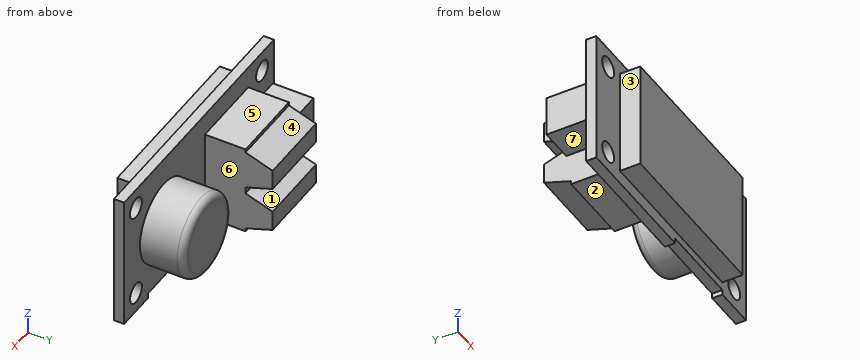
from build123d import *

# Parameters (mm, degrees)
SKETCH1_R           = 1.5
BOSS_EXTRUDE1_DEPTH = 1.5
SKETCH2_R           = 6
BOSS_EXTRUDE2_DEPTH = 6.5
FILLET1_R           = 1
SKETCH3_W           = 5
SKETCH3_H           = 6
BOSS_EXTRUDE3_DEPTH = 6
BOSS_EXTRUDE4_START = -12.5
BOSS_EXTRUDE4_DEPTH = 11
SKETCH6_W           = 26
SKETCH6_H           = 16
BOSS_EXTRUDE5_DEPTH = 3


with BuildPart() as part:
    # Sketch1 → Boss-Extrude1 (new body)
    with BuildSketch(Plane(origin=(0, 0, 0), x_dir=(1, 0, 0), z_dir=(0, 1, 0))):
        Polygon((-19, -10), (19, -10), (19, 10), (13, 10), (13, 9.25), (1, 9.25), (1, 10), (-19, 10), align=None)
        with Locations((-16, 7)):
            Circle(SKETCH1_R, mode=Mode.SUBTRACT)
        with Locations((-16, -7)):
            Circle(SKETCH1_R, mode=Mode.SUBTRACT)
        with Locations((16, -7)):
            Circle(SKETCH1_R, mode=Mode.SUBTRACT)
        with Locations((16, 7)):
            Circle(SKETCH1_R, mode=Mode.SUBTRACT)
    extrude(amount=BOSS_EXTRUDE1_DEPTH)

    # Sketch2 → Boss-Extrude2 (add)
    with BuildSketch(Plane(origin=(0, 1.5, 0), x_dir=(1, 0, 0), z_dir=(0, 1, 0))):
        with Locations((9, 0)):
            Circle(SKETCH2_R)
    extrude(amount=BOSS_EXTRUDE2_DEPTH)

    # Fillet1
    fillet1_edges = [part.edges().sort_by_distance(p)[0] for p in [
        (3, 8, 0),
    ]]
    fillet(fillet1_edges, radius=FILLET1_R)

    # Sketch3 → Boss-Extrude3 (add)
    with BuildSketch(Plane(origin=(0, 1.5, 0), x_dir=(1, 0, 0), z_dir=(0, 1, 0))):
        with Locations((-16.25, 0)):
            Rectangle(SKETCH3_W, SKETCH3_H)
    extrude(amount=BOSS_EXTRUDE3_DEPTH)

    # Sketch5 → Boss-Extrude4 (add)
    with BuildSketch(Plane(origin=(0, 0, 0), x_dir=(0, 0, -1), z_dir=(1, 0, 0)).offset(BOSS_EXTRUDE4_START)):
        Polygon((6.75, 1.5), (6.75, 7.5), (6.25, 7.5), (4.875, 11.5), (1.875, 11.5), (0.5, 7.5), (-0.5, 7.5), (-1.875, 11.5), (-4.875, 11.5), (-6.25, 7.5), (-6.75, 7.5), (-6.75, 1.5), align=None)
    extrude(amount=BOSS_EXTRUDE4_DEPTH)

    # Sketch6 → Boss-Extrude5 (add)
    with BuildSketch(Plane.XZ):
        Rectangle(SKETCH6_W, SKETCH6_H)
    extrude(amount=BOSS_EXTRUDE5_DEPTH)


solid = part.part
Read the model definition and answer for the solid it produces. Units are mm, in the model's axes. Face numbers are marked on the shaded views. A direction names the side the tool comes from. Give positions to 0.01 mm unless a question says otherwise; leave off trailing zeros. Write each loop counter-clockwise with the first axis right and the second up, starting at its lowest first coordinate (ties: lowest second). Pieces come first, ordered by that corner, then holes. Notation, with made-up numbers: (47.25, 11.25) - (64.25, 11.25) arc R27 cw to (64.25, 33.25) - close; hole circle Ø7 at (1.25, -7.75). An arc over 180 degrees is marked (long way). Return JSON: item names as keys, results as strings.
Q1. For a pull along Z with two mould halves and no side action, classify the marked faces 1, 2, 3 and 4 as released by +Z, released by -Z, zero draft, split by the parting line, or undercut.
Reply:
{"face 1": "undercut", "face 2": "released by -Z", "face 3": "zero draft", "face 4": "released by +Z"}
Q2. A cutting plane is placed at D-D, the plane x = 9. Determine the outline of the cut face in (y, z).
Reply:
{"outline": "(-3, -8) - (0, -8) - (0, -9.25) - (1.5, -9.25) - (1.5, -6) - (7, -6) arc R1 ccw to (8, -5) - (8, 5) arc R1 ccw to (7, 6) - (1.5, 6) - (1.5, 10) - (0, 10) - (0, 8) - (-3, 8) - close"}
Q3. A cutting plane is placed at B-B, the plane y = 4.25. Determine the outline of the cut face in (x, z).
Reply:
{"outline": "(-18.75, -3) - (-13.75, -3) - (-13.75, 3) - (-18.75, 3) - close; (-12.5, -6.75) - (-1.5, -6.75) - (-1.5, 6.75) - (-12.5, 6.75) - close; circle Ø12 at (9, 0)"}
Q4. Given P1, Ø2.5, axis at x = 1, y = -2, coming from the +Z side; P2, Ø2.5, axis at y = -2, z = 0.5, coming from the -X side; P3, Ø1.5, axis at x = -15.5, y = 3.5, coming from the -Z side, each flat-ended and moving along its own axis, determine where each tip first touches the part or whether it passes through.
Reply:
{"P1": "z = 8", "P2": "x = -13", "P3": "z = -3"}
Q5. A cutting plane is placed at A-A, the plane x = 16. Determine the outline of the cut face in (y, z).
Reply:
{"outline": "(0, -10) - (1.5, -10) - (1.5, -8.5) - (0, -8.5) - close; (0, -5.5) - (1.5, -5.5) - (1.5, 5.5) - (0, 5.5) - close; (0, 8.5) - (1.5, 8.5) - (1.5, 10) - (0, 10) - close"}
Q6. Consider line 1 along X through (y, z) = (0.75, 7); line 2 along Z through (x, y) = (16, 1.2); line 3 along Y through (x, z) = (14.5, 3.5). Determine where each line is inside the solid, lowest interval first. Write a range as [from, to].
Reply:
{"line 1": "[-19, -17.5], [-14.5, 14.5], [17.5, 19]", "line 2": "[-10, -8.5], [-5.5, 5.5], [8.5, 10]", "line 3": "[0, 1.5]"}
Q7. For the marked faces 5, 6 and 7, determine the directions among +Z, -Z, +X, -X, +Y, -Y from which every point of the face is accessible in a straight line to the end or side of a thin tool.
Reply:
{"face 5": "+Z, +X, -X, +Y", "face 6": "+Z, -Z, +Y", "face 7": "-Z, -X, +Y"}
Q8. A cutting plane is placed at C-C, the plane z = 0. Determine the outline of the cut face in (x, y).
Reply:
{"outline": "(-19, 0) - (-13, 0) - (-13, -3) - (13, -3) - (13, 0) - (19, 0) - (19, 1.5) - (15, 1.5) - (15, 7) arc R1 ccw to (14, 8) - (4, 8) arc R1 ccw to (3, 7) - (3, 1.5) - (-1.5, 1.5) - (-1.5, 7.5) - (-12.5, 7.5) - (-12.5, 1.5) - (-13.75, 1.5) - (-13.75, 7.5) - (-18.75, 7.5) - (-18.75, 1.5) - (-19, 1.5) - close"}
